Could you check a few things on this model? Use its own coordinates, in mm. Face numbers are marked on the shaded views. Give positions to 0.01 mm unless a question says otherwise; leave off trailing zeros. Loops run counter-clockwise (first coordinate to the right, second up) from the corner with the lowest first, then second, coordinate; pieces in that order, holes last. Notation, with made-up numbers: M -30,15 L -9,15 A12 cw -9,27 Z; hole C 35,1.25 d10. An arc over 180 degrees is marked long. Return JSON: item names as keys, results as strings. Group by question number.
1. If we section it at C-C (x = 30): Write out the boundary of the cut face in (y, z), plus the area to 3 significant figures.
2. If we section it at B-B (y = -6): Write out the boundary of the cut face in (x, z), plus the area to 3 significant figures.
3. If we mould it in two halves opening along Y, with no side actions, what happens to the marked faces 1, 2, 3 and 4? For each: +Y half, -Y half, draft (parallel to the pull), parting line (faces both ways), or undercut.
4. If we section it at D-D (z = 67): Write out the boundary of the cut face in (x, y), plus the area to 3 significant figures.
5. Please list where these lines run through material, in increasing order: line 1 (Y direction, x = 29.5, z = 31); line 2 (X direction, y = -10, z = 29); line 3 (Z direction, x = 25.5, y = -11).
6. If we section it at A-A (z = 32): Write out the boundary of the cut face in (x, y).
7. For pin 1 (2 mm diameter, centred on x = 25, y = -9, fed in from +Z); pin 2 (4 mm diameter, centred on y = -3, z = 74.5, fed in from -X); pin 3 (5 mm diameter, centred on y = -9.5, z = 74.5, fed in from -X); pin 4 (8 mm diameter, centred on x = 9.5, z = 55.5, fed in from -Y), each with a flat end and sliding along its axis, tell me the tip position at first contact or that it passes through.
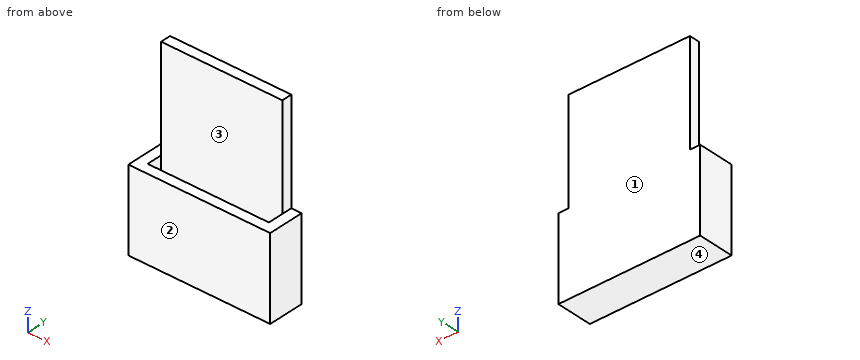
```python
from build123d import *

# Parameters (mm, degrees)
F1_DEPTH = 59
F2_W     = 17.5
F2_H     = 40
F3_DEPTH = 5
F4_W     = 17.5
F4_H     = 40
F5_DEPTH = 5


with BuildPart() as f1:
    # F0 (on Right) → F1 (new body)
    with BuildSketch(Plane.YZ):
        Polygon((-17.5, 0), (0, 0), (0, 90), (-5, 90), (-5, 8), (-12.5, 8), (-12.5, 40), (-17.5, 40), align=None)
    extrude(amount=F1_DEPTH)

    # F2 (on face) → F3 (join)
    with BuildSketch(Plane.YZ.offset(59)):
        with Locations((-8.75, 20)):
            Rectangle(F2_W, F2_H)
    extrude(amount=F3_DEPTH)

    # F4 (on face) → F5 (join)
    with BuildSketch(Plane(origin=(0, 0, 0), x_dir=(0, -1, 0), z_dir=(-1, 0, 0))):
        with Locations((8.75, 20)):
            Rectangle(F4_W, F4_H)
    extrude(amount=F5_DEPTH)


solid = f1.part
```
Answer:
{
 "1": {"outline": "M -17.5,0 L 0,0 L 0,90 L -5,90 L -5,8 L -12.5,8 L -12.5,40 L -17.5,40 Z", "area": "710 mm²"},
 "2": {"outline": "M -5,0 L 64,0 L 64,40 L 59,40 L 59,8 L 0,8 L 0,40 L -5,40 Z", "area": "872 mm²"},
 "3": {"face 1": "+Y half", "face 2": "-Y half", "face 3": "undercut", "face 4": "draft"},
 "4": {"outline": "M 0,-5 L 59,-5 L 59,0 L 0,0 Z", "area": "295 mm²"},
 "5": {"line 1": "y = -17.5 to -12.5, -5 to 0", "line 2": "x = -5 to 0, 59 to 64", "line 3": "z = 0 to 8"},
 "6": {"outline": "M -5,-17.5 L 64,-17.5 L 64,0 L -5,0 Z; hole M 0,-12.5 L 59,-12.5 L 59,-5 L 0,-5 Z"},
 "7": {"pin 1": "stops at z = 8", "pin 2": "stops at x = 0", "pin 3": "passes through", "pin 4": "stops at y = -5"}
}
